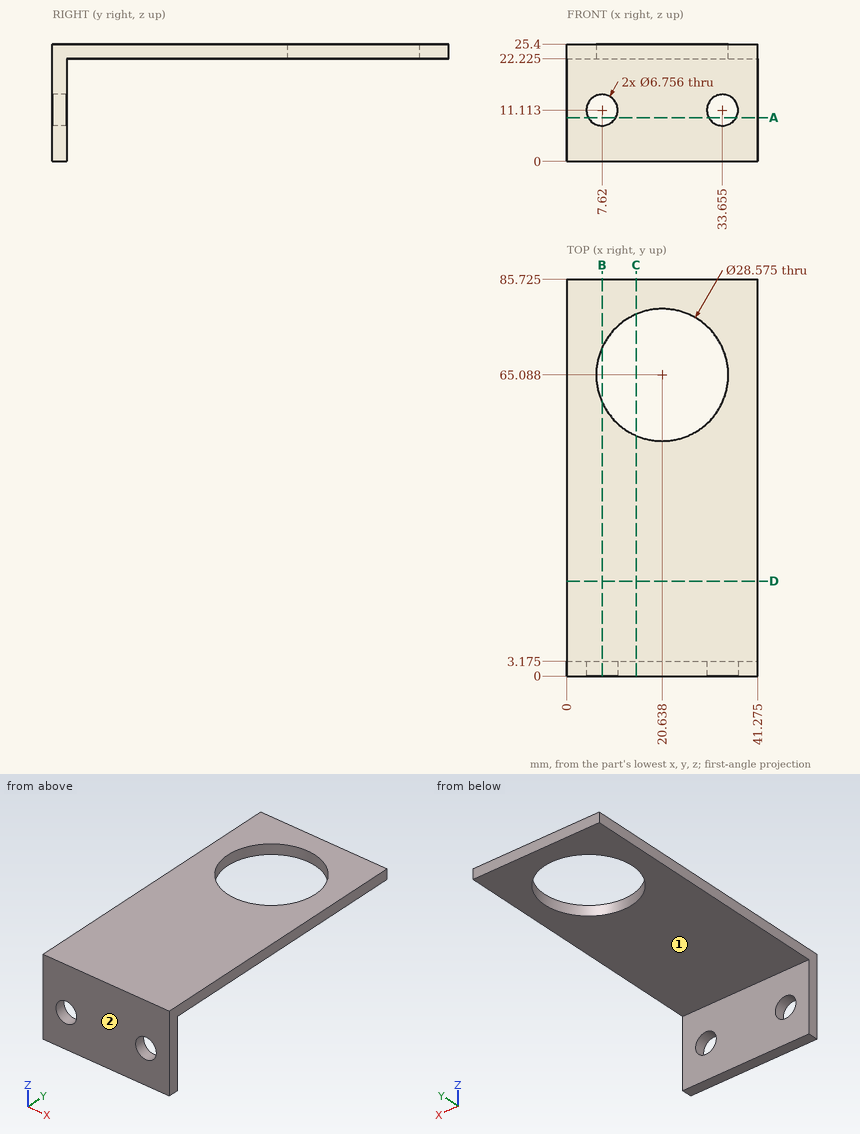
Answer from the drawing. Dimensions are ordinates in mm from the lowest x, y and z of the part. A direction names the side the tool comes from. Round coordinates to 2 decimals unless told otherwise and drop trailing zeros. Loops run counter-clockwise (first coordinate to the right, second up) from the corner with the lowest first, then second, coordinate; pieces in that order, holes last.
(1) The part is cut by section D-D, the plane y = 20.5. Give the vertices of the cut face in (x, z) (1 decimal).
Computed values:
outline: (0, 22.2) - (41.3, 22.2) - (41.3, 25.4) - (0, 25.4) - close
(2) The part is cut by section C-C, the plane x = 15. Give the vertices of the cut face in (y, z) (1 decimal).
Computed values:
outline: (0, 0) - (3.2, 0) - (3.2, 22.2) - (52, 22.2) - (52, 25.4) - (0, 25.4) - close; (78.2, 22.2) - (85.7, 22.2) - (85.7, 25.4) - (78.2, 25.4) - close
(3) Each of these flat-tipped pins is pushed along its axis until it touches: P1, Ø5, axis at x = 8, y = 56.5, coming from the -Z side (1 decimal); P2, Ø2, axis at x = 29.5, z = 5, coming from the +Y side (1 decimal). Where does it stop, or does it pass through?
Computed values:
P1: stops at z = 22.2
P2: stops at y = 3.2
(4) The part is cut by section A-A, the plane z = 9.5. Give the vertices of the cut face in (x, y) (1 decimal).
Computed values:
outline: (0, 0) - (4.7, 0) - (4.7, 3.2) - (0, 3.2) - close; (10.6, 0) - (30.7, 0) - (30.7, 3.2) - (10.6, 3.2) - close; (36.6, 0) - (41.3, 0) - (41.3, 3.2) - (36.6, 3.2) - close
(5) For the marked faces 1 and 2, determine the directions among +Z, -Z, +X, -X, +Y, -Y from which every point of the face is accessible in a straight line to the end or side of a thin tool.
Computed values:
face 1: -Z, +X, -X, +Y
face 2: +Z, -Z, +X, -X, -Y
(6) Find the intervals of material crossed by L1, parallel to Z at x = 7.62, y = 1.45 (1 decimal); L2, parallel to Y at x = 38, z = 4.25 (1 decimal); L3, parallel to Z at x = 5.5, y = 57 (1 decimal), in increasing order.
Computed values:
L1: z = 0 to 7.7, 14.5 to 25.4
L2: y = 0 to 3.2
L3: z = 22.2 to 25.4
(7) The part is cut by section B-B, the plane x = 7.62. Give the vertices of the cut face in (y, z) (1 decimal), and give its area (3 significant figures).
Computed values:
outline: (0, 0) - (3.2, 0) - (3.2, 7.7) - (0, 7.7) - close; (0, 14.5) - (3.2, 14.5) - (3.2, 22.2) - (59.2, 22.2) - (59.2, 25.4) - (0, 25.4) - close; (71, 22.2) - (85.7, 22.2) - (85.7, 25.4) - (71, 25.4) - close
area: 284 mm2
